```python
from build123d import *

# Parameters (mm, degrees)
BOSS_EXTRUDE1_DEPTH     = 193.4
CUT_EXTRUDE1_DEPTH      = 38
CUT_EXTRUDE1_DEPTH_BACK = 38
BOSS_EXTRUDE2_DEPTH     = 4.5
CUT_EXTRUDE2_DEPTH      = 40
CUT_EXTRUDE3_DEPTH      = 42
CUT_EXTRUDE4_DEPTH      = 81.5
CUT_EXTRUDE5_DEPTH      = 81.5
SKETCH8_W               = 2
SKETCH8_H               = 108
CUT_EXTRUDE6_DEPTH      = 4
SKETCH9_W               = 2.75
SKETCH9_H               = 4
LPATTERN1_COUNT         = 2
LPATTERN1_PITCH         = 20
LPATTERN1_COUNT_DIR2    = 2
LPATTERN1_PITCH_DIR2    = 18
LPATTERN2_COUNT         = 2
LPATTERN2_PITCH         = 38
LPATTERN2_COUNT_DIR2    = 2
LPATTERN2_PITCH_DIR2    = 38


with BuildPart() as part:
    # Sketch1 → Boss-Extrude1 (new body)
    with BuildSketch(Plane.XY.offset(-193.4)):
        with BuildLine():
            Line((-38, 58.5), (-38, 4.5))
            Line((-38, 4.5), (-24.503877244, 4.5))
            ThreePointArc((-24.503877244, 4.5), (0, 1.1), (24.503877244, 4.5))
            Line((24.503877244, 4.5), (38, 4.5))
            Line((38, 4.5), (38, 58.5))
            Line((38, 58.5), (24.503877244, 58.5))
            ThreePointArc((24.503877244, 58.5), (0, 61.9), (-24.503877244, 58.5))
            Line((-24.503877244, 58.5), (-38, 58.5))
        make_face()
    extrude(amount=BOSS_EXTRUDE1_DEPTH)

    # Sketch2 → Cut-Extrude1 (cut, two sides)
    with BuildSketch(Plane(origin=(0, 0, 0), x_dir=(0, 0, -1), z_dir=(1, 0, 0))) as cut_extrude1_sk:
        with BuildLine():
            Line((0, -5), (189.4, -5))
            Line((189.4, -5), (189.4, 4.5))
            Line((189.4, 4.5), (49, 4.5))
            ThreePointArc((49, 4.5), (46.878679656, 5.378679656), (46, 7.5))
            Line((46, 7.5), (46, 13.5))
            ThreePointArc((46, 13.5), (45.121320344, 15.621320344), (43, 16.5))
            Line((43, 16.5), (37, 16.5))
            ThreePointArc((37, 16.5), (35.585786438, 15.914213562), (35, 14.5))
            Line((35, 14.5), (35, 0))
            Line((35, 0), (5, 0))
            Line((5, 0), (5, 31.5))
            ThreePointArc((5, 31.5), (9.393398282, 42.106601718), (20, 46.5))
            Line((20, 46.5), (43, 46.5))
            ThreePointArc((43, 46.5), (45.121320344, 47.378679656), (46, 49.5))
            Line((46, 49.5), (46, 55.5))
            ThreePointArc((46, 55.5), (46.878679656, 57.621320344), (49, 58.5))
            Line((49, 58.5), (189.4, 58.5))
            Line((189.4, 58.5), (189.4, 63.5))
            Line((189.4, 63.5), (0, 63.5))
            Line((0, 63.5), (0, -5))
        make_face()
    extrude(amount=CUT_EXTRUDE1_DEPTH, mode=Mode.SUBTRACT)
    extrude(cut_extrude1_sk.sketch, amount=-CUT_EXTRUDE1_DEPTH_BACK, mode=Mode.SUBTRACT)

    # Sketch3 → Boss-Extrude2 (add)
    with BuildSketch(Plane(origin=(0, 0, 0), x_dir=(1, 0, 0), z_dir=(0, 1, 0))):
        with BuildLine():
            Line((-38, 5), (-21.865, 5))
            ThreePointArc((-21.865, 5), (-21.226384959, 4.895302306), (-20.654631441, 4.59217083))
            Line((-20.654631441, 4.59217083), (-15.150368559, 0.40782917))
            ThreePointArc((-15.150368559, 0.40782917), (-14.578615041, 0.104697694), (-13.94, 0))
            Line((-13.94, 0), (13.94, 0))
            ThreePointArc((13.94, 0), (14.578615041, 0.104697694), (15.150368559, 0.40782917))
            Line((15.150368559, 0.40782917), (20.654631441, 4.59217083))
            ThreePointArc((20.654631441, 4.59217083), (21.226384959, 4.895302306), (21.865, 5))
            Line((21.865, 5), (38, 5))
            Line((38, 5), (38, 35))
            Line((38, 35), (21.865, 35))
            ThreePointArc((21.865, 35), (21.226384959, 35.104697694), (20.654631441, 35.40782917))
            Line((20.654631441, 35.40782917), (15.150368559, 39.59217083))
            ThreePointArc((15.150368559, 39.59217083), (14.578615041, 39.895302306), (13.94, 40))
            Line((13.94, 40), (-13.94, 40))
            ThreePointArc((-13.94, 40), (-14.578615041, 39.895302306), (-15.150368559, 39.59217083))
            Line((-15.150368559, 39.59217083), (-20.654631441, 35.40782917))
            ThreePointArc((-20.654631441, 35.40782917), (-21.226384959, 35.104697694), (-21.865, 35))
            Line((-21.865, 35), (-38, 35))
            Line((-38, 35), (-38, 5))
        make_face()
    extrude(amount=BOSS_EXTRUDE2_DEPTH)

    # Sketch4 → Cut-Extrude2 (cut)
    with BuildSketch(Plane.XY):
        with BuildLine():
            Line((-38, -5), (38, -5))
            Line((38, -5), (38, 8))
            ThreePointArc((38, 8), (35.656854249, 2.343145751), (30, 0))
            Line((30, 0), (-30, 0))
            ThreePointArc((-30, 0), (-35.656854249, 2.343145751), (-38, 8))
            Line((-38, 8), (-38, -5))
        make_face()
    extrude(amount=-CUT_EXTRUDE2_DEPTH, mode=Mode.SUBTRACT)

    # Sketch5 → Cut-Extrude3 (cut)
    with BuildSketch(Plane.XY):
        with BuildLine():
            Line((-31, 4), (31, 4))
            ThreePointArc((31, 4), (33.121320344, 4.878679656), (34, 7))
            Line((34, 7), (34, 62))
            Line((34, 62), (-34, 62))
            Line((-34, 62), (-34, 7))
            ThreePointArc((-34, 7), (-33.121320344, 4.878679656), (-31, 4))
        make_face()
    extrude(amount=-CUT_EXTRUDE3_DEPTH, mode=Mode.SUBTRACT)

    # Sketch6 → Cut-Extrude4 (cut)
    with BuildSketch(Plane(origin=(0, 0, 0), x_dir=(1, 0, 0), z_dir=(0, 1, 0))):
        with BuildLine():
            Line((-34, 186.4), (-34, 41))
            Line((-34, 41), (34, 41))
            Line((34, 41), (34, 186.4))
            ThreePointArc((34, 186.4), (33.121320344, 188.521320344), (31, 189.4))
            Line((31, 189.4), (-31, 189.4))
            ThreePointArc((-31, 189.4), (-33.121320344, 188.521320344), (-34, 186.4))
        make_face()
    extrude(amount=CUT_EXTRUDE4_DEPTH, mode=Mode.SUBTRACT)

    # Sketch7 → Cut-Extrude5 (cut)
    with BuildSketch(Plane(origin=(0, 0, 0), x_dir=(1, 0, 0), z_dir=(0, 1, 0))):
        with BuildLine():
            Line((-32, 193.4), (32, 193.4))
            ThreePointArc((32, 193.4), (36.242640687, 191.642640687), (38, 187.4))
            Line((38, 187.4), (38, 198.4))
            Line((38, 198.4), (-38, 198.4))
            Line((-38, 198.4), (-38, 187.4))
            ThreePointArc((-38, 187.4), (-36.242640687, 191.642640687), (-32, 193.4))
        make_face()
    extrude(amount=CUT_EXTRUDE5_DEPTH, mode=Mode.SUBTRACT)

    # Sketch8 → Cut-Extrude6 (cut)
    with BuildSketch(Plane.XY.offset(-193.4)):
        with Locations((0, 54)):
            Rectangle(SKETCH8_W, SKETCH8_H)
    extrude(amount=CUT_EXTRUDE6_DEPTH, mode=Mode.SUBTRACT)

    # Sketch9 → Cut-Revolve1 (revolve, cut)
    with BuildSketch(Plane(origin=(9, 0, 0), x_dir=(0, 0, -1), z_dir=(1, 0, 0))):
        with Locations((11.375, 2)):
            Rectangle(SKETCH9_W, SKETCH9_H)
    cut_revolve1 = revolve(axis=Axis((9, 0, -10), (0, 1, 0)), mode=Mode.SUBTRACT)

    # LPattern1: Cut-Revolve1 2 × 2
    with Locations(*[(-j * LPATTERN1_PITCH_DIR2, 0, -i * LPATTERN1_PITCH) for i in range(LPATTERN1_COUNT) for j in range(LPATTERN1_COUNT_DIR2) if (i, j) != (0, 0)]):
        add(cut_revolve1, mode=Mode.SUBTRACT)

    # Sketch11 → Cut-Revolve2 (revolve, cut)
    with BuildSketch(Plane(origin=(19, 0, 0), x_dir=(0, 0, -1), z_dir=(1, 0, 0))):
        Polygon((189.4, 12.5), (189.4, 14.9585), (192.8585, 14.9585), (193.4, 15.5), (193.4, 12.5), align=None)
    cut_revolve2 = revolve(axis=Axis((19, 12.5, -193.4), (0, 0, 1)), mode=Mode.SUBTRACT)

    # LPattern2: Cut-Revolve2 2 × 2
    with Locations(*[(-j * LPATTERN2_PITCH_DIR2, i * LPATTERN2_PITCH, 0) for i in range(LPATTERN2_COUNT) for j in range(LPATTERN2_COUNT_DIR2) if (i, j) != (0, 0)]):
        add(cut_revolve2, mode=Mode.SUBTRACT)


solid = part.part
```
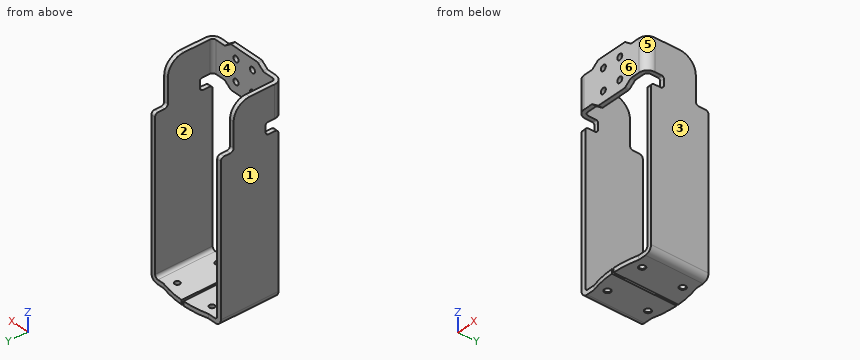
Part model, mm, in its own coordinate system. Face numbers are marked on the shaded views. A direction names the side the tool comes from. Give positions to 0.01 mm unless a question says otherwise; leave off trailing zeros. Write each loop counter-clockwise with the first axis right and the second up, starting at its lowest first coordinate (ties: lowest second). Pieces come first, ordered by that corner, then holes. Notation, with made-up numbers: (8.25, 10.5) -> (28.25, 10.5) arc R26 ccw to (28.25, 28.5) -> close; hole circle Ø4 at (-32.75, 34). An arc over 180 degrees is marked (long way). Put each result on its own line as item: value. Start each with the question number.
Item 1: Cut at A-A (z = -30). List the corners of the cut face in (x, y), then the cut area to 3 significant figures.
Item 2: Cut at C-C (z = -77). List the corners of the cut face in (x, y), then the cut area to 3 significant figures.
Item 3: Cut at B-B (x = -26.5). List the corners of the cut face in (y, z), then the cut area to 3 significant figures.
Item 4: Cut at D-D (y = 43). List the corners of the cut face in (x, z).
Item 5: Which spindle directions (+Z, -Z, +X, -X, +Y, -Y) get a long thin tool onto all of the face, cutting with end or side? Do the marked faces 4, 5 and 6. Say none if no direction does.
Item 6: Wall check: L1, parallel to Z at x = -9, y = 1.3; L2, parallel to X at y = 37, z = -31.5; L3, parallel to Z at x = -9, y = 3.1. Give the ranges that are in metal, low to high. Write a range as [from, to].
Item 7: Pin check, flat tips, straight feed: pin 1 Ø3 at (x, y) = (-19, 12.5) entering from -Z; pin 2 Ø2 at (x, y) = (36, 53) entering from +Z; pin 3 Ø11 at (x, z) = (-29, -122) entering from -Y; pin 4 Ø6.5 at (x, z) = (9, -10) entering from -Y. Stop position of each tip, or through.
Item 8: Pull direction X, two halves, no side cores. Call the marked faces 1, 2 and 3: pulls with the +X half, pulls with the -X half, needs draft (parallel to the pull), parting line crosses it, or undercut.
Answer list:
1. outline: (-38, 8) arc R8 ccw to (-30, 0) -> (-11.75, 0) -> (-11.75, 4) -> (-31, 4) arc R3 cw to (-34, 7) -> (-34, 46.5) -> (-38, 46.5) -> close; (-6.25, 0) -> (6.25, 0) -> (6.25, 4) -> (-6.25, 4) -> close; (11.75, 0) -> (30, 0) arc R8 ccw to (38, 8) -> (38, 46.5) -> (34, 46.5) -> (34, 7) arc R3 cw to (31, 4) -> (11.75, 4) -> close
1. area: 576 mm2
2. outline: (-38, 4.5) -> (-34, 4.5) -> (-34, 58.5) -> (-38, 58.5) -> close; (34, 4.5) -> (38, 4.5) -> (38, 58.5) -> (34, 58.5) -> close
2. area: 432 mm2
3. outline: (0, -35) -> (4, -35) -> (4, -5) -> (0, -5) -> close; (4.5, -193.4) -> (58.5, -193.4) -> (58.5, -189.4) -> (4.5, -189.4) -> close
3. area: 336 mm2
4. outline: (-38, -187.4) arc R6 ccw to (-32, -193.4) -> (-1, -193.4) -> (-1, -189.4) -> (-31, -189.4) arc R3 cw to (-34, -186.4) -> (-34, -10.37) -> (-38, -10.37) -> close; (1, -193.4) -> (32, -193.4) arc R6 ccw to (38, -187.4) -> (38, -10.37) -> (34, -10.37) -> (34, -186.4) arc R3 cw to (31, -189.4) -> (1, -189.4) -> close
5. face 4: +Z, +Y
5. face 5: +Z, +X, -Y
5. face 6: +Z, -Z, +X, -X, -Y
6. L1: z = [-40, -32.75], [-27.25, -12.75], [-7.25, 0]
6. L2: x = [-38, -34], [34, 38]
6. L3: z = [-193.4, -189.4], [-40, -32.75], [-27.25, -12.75], [-7.25, 0]
7. pin 1: passes through
7. pin 2: stops at z = -46
7. pin 3: stops at y = 4.5
7. pin 4: stops at y = 0
8. face 1: pulls with the -X half
8. face 2: undercut
8. face 3: pulls with the +X half
